from build123d import *

# Parameters (mm, degrees)
BOSS_EXTRUDE1_DEPTH                       = 3.175
CSK_FOR_0_FLAT_HEAD_MACHINE_SCREW_2_COUNT = 2
CSK_FOR_0_FLAT_HEAD_MACHINE_SCREW_2_PITCH = 47.625
LPATTERN1_COUNT                           = 4
LPATTERN1_PITCH                           = 25.4
LPATTERN2_COUNT                           = 3
LPATTERN2_PITCH                           = 50.8


with BuildPart() as part:
    # Sketch1 → Boss-Extrude1 (new body)
    with BuildSketch(Plane.XY):
        with BuildLine():
            Line((0, 0), (0, 220.98))
            Line((0, 220.98), (-6.35, 220.98))
            ThreePointArc((-6.35, 220.98), (-10.840128061, 222.839871939), (-12.7, 227.33))
            Line((-12.7, 227.33), (-12.7, 284.48))
            Line((-12.7, 284.48), (-129.54, 284.48))
            Line((-129.54, 284.48), (-129.54, 227.33))
            Line((-129.54, 227.33), (-44.45, 0))
            Line((-44.45, 0), (0, 0))
        make_face()
    extrude(amount=-BOSS_EXTRUDE1_DEPTH)

    # Sketch3 → CSK for _0 Flat Head Machine Screw _100 (revolve, cut)
    with BuildSketch(Plane(origin=(-114.3, 278.13, 0), x_dir=(0, -1, 0), z_dir=(1, 0, 0))):
        Polygon((0, 0), (0, 3.175), (2.7559, 3.175), (2.7559, 2.4384), (5.1943, 0), align=None)
    csk_for_0_flat_head_machine_screw_100 = revolve(axis=Axis((-114.3, 278.13, 6.35), (0, 0, -1)), mode=Mode.SUBTRACT)

    # CSK for _0 Flat Head Machine Screw _ 2: CSK for _0 Flat Head Machine Screw _100 ×2
    with Locations(*[(0, -i * CSK_FOR_0_FLAT_HEAD_MACHINE_SCREW_2_PITCH, 0) for i in range(1, CSK_FOR_0_FLAT_HEAD_MACHINE_SCREW_2_COUNT)]):
        add(csk_for_0_flat_head_machine_screw_100, mode=Mode.SUBTRACT)

    # LPattern1: CSK for _0 Flat Head Machine Screw _100 ×4
    with Locations(*[(i * LPATTERN1_PITCH, 0, 0) for i in range(1, LPATTERN1_COUNT)]):
        add(csk_for_0_flat_head_machine_screw_100, mode=Mode.SUBTRACT)

    # LPattern1 copy 1 sketch → LPattern1 copy 1 (revolve, cut)
    with BuildSketch(Plane(origin=(-88.9, 230.505, 0), x_dir=(0, -1, 0), z_dir=(1, 0, 0))):
        Polygon((0, 0), (0, 3.175), (2.7559, 3.175), (2.7559, 2.4384), (5.1943, 0), align=None)
    revolve(axis=Axis((-88.9, 230.505, 6.35), (0, 0, -1)), mode=Mode.SUBTRACT)

    # LPattern1 copy 2 sketch → LPattern1 copy 2 (revolve, cut)
    with BuildSketch(Plane(origin=(-63.5, 230.505, 0), x_dir=(0, -1, 0), z_dir=(1, 0, 0))):
        Polygon((0, 0), (0, 3.175), (2.7559, 3.175), (2.7559, 2.4384), (5.1943, 0), align=None)
    revolve(axis=Axis((-63.5, 230.505, 6.35), (0, 0, -1)), mode=Mode.SUBTRACT)

    # LPattern1 copy 3 sketch → LPattern1 copy 3 (revolve, cut)
    with BuildSketch(Plane(origin=(-38.1, 230.505, 0), x_dir=(0, -1, 0), z_dir=(1, 0, 0))):
        Polygon((0, 0), (0, 3.175), (2.7559, 3.175), (2.7559, 2.4384), (5.1943, 0), align=None)
    revolve(axis=Axis((-38.1, 230.505, 6.35), (0, 0, -1)), mode=Mode.SUBTRACT)

    # Sketch4 → CSK for _0 Flat Head Machine Screw _ 3 (revolve, cut)
    with BuildSketch(Plane(origin=(-15.875, 107.95, 0), x_dir=(0, -1, 0), z_dir=(1, 0, 0))):
        Polygon((0, 0), (0, 3.175), (2.7559, 3.175), (2.7559, 2.4384), (5.1943, 0), align=None)
    csk_for_0_flat_head_machine_screw_3 = revolve(axis=Axis((-15.875, 107.95, 6.35), (0, 0, -1)), mode=Mode.SUBTRACT)

    # LPattern2: CSK for _0 Flat Head Machine Screw _ 3 ×3
    with Locations(*[(0, -i * LPATTERN2_PITCH, 0) for i in range(1, LPATTERN2_COUNT)]):
        add(csk_for_0_flat_head_machine_screw_3, mode=Mode.SUBTRACT)


solid = part.part
The listing builds one solid part. Answer for the finished solid, in the listing's coordinates (mm). Round coordinates to 2 decimals unless told otherwise and drop trailing zeros. Write each loop counter-clockwise with the first axis right and the second up, starting at its lowest first coordinate (ties: lowest second). Pieces come first, ordered by that corner, then holes. Notation, with made-up numbers: (32, -22) - (67, -22) arc R35 cw to (67, 14) - close; hole circle Ø10 at (-16.5, 39). An arc over 180 degrees is marked (long way). Use a Markdown table: item, result. Add a question column.
1. The part is cut by section C-C (y = 6.35). Write down the section's boundary in (x, z) (3 decimals).
2. The part is cut by section A-A (y = 278.13). Write down the section's boundary in (x, z) (3 decimals), and give its area (3 significant figures).
3. The part is cut by section B-B (x = -38.1). Write down the section's boundary in (y, z) (3 decimals), and give its area (3 significant figures).
4. Flat-ended cylindrical pins translate along their axes: P1, Ø6.5, axis at x = -63.5, y = 230.505, coming from the -Z side (3 decimals); P2, Ø4.5, axis at x = -114.3, y = 230.505, coming from the -Z side; P3, Ø9, axis at x = -114.3, y = 278.13, coming from the +Z side; P4, Ø1, axis at x = -4, z = -1.5, coming from the +Y side. Find the tip coordinate at first contact, or state that the pin passes through.
5. Consider line 1 (X direction, y = 278.13, z = -2.65); line 2 (X direction, y = 228, z = -0.5); line 3 (X direction, y = 234.5, z = -2). Determine where each line is inside the solid, lowest interval first.
6. The part is cut by section D-D (z = -1.55). Give the number of separate pieces and of enclosed holes in the cut face, and give its area (3 significant figures).
7. For a pull along Y with two mould halves and no side action, classify faces 1 (the face through (-38.221, 280.883, -2.802)), 2 (the face through (-10.8, 222.8, -1.6)), 3 (the face through (-87.59, 115.26, -1.57)) as +Y half, -Y half, draft (parallel to the pull), parting line (faces both ways), or undercut.
Reported:
| question | item | result |
|---|---|---|
| 1 | outline | (-46.827, -3.175) - (-18.631, -3.175) - (-18.631, -2.438) - (-21.069, 0) - (-46.827, 0) - close; (-13.119, -3.175) - (0, -3.175) - (0, 0) - (-10.681, 0) - (-13.119, -2.438) - close |
| 2 | outline | (-129.54, -3.175) - (-117.056, -3.175) - (-117.056, -2.438) - (-119.494, 0) - (-129.54, 0) - close; (-111.544, -3.175) - (-91.656, -3.175) - (-91.656, -2.438) - (-94.094, 0) - (-109.106, 0) - (-111.544, -2.438) - close; (-86.144, -3.175) - (-66.256, -3.175) - (-66.256, -2.438) - (-68.694, 0) - (-83.706, 0) - (-86.144, -2.438) - close; (-60.744, -3.175) - (-40.856, -3.175) - (-40.856, -2.438) - (-43.294, 0) - (-58.306, 0) - (-60.744, -2.438) - close; (-35.344, -3.175) - (-12.7, -3.175) - (-12.7, 0) - (-32.906, 0) - (-35.344, -2.438) - close |
| 2 | area | 277 mm^2 |
| 3 | outline | (0, -3.175) - (227.749, -3.175) - (227.749, -2.438) - (225.311, 0) - (0, 0) - close; (233.261, -3.175) - (275.374, -3.175) - (275.374, -2.438) - (272.936, 0) - (235.699, 0) - (233.261, -2.438) - close; (280.886, -3.175) - (284.48, -3.175) - (284.48, 0) - (283.324, 0) - (280.886, -2.438) - close |
| 3 | area | 856 mm^2 |
| 4 | P1 | z = -3.175 |
| 4 | P2 | through |
| 4 | P3 | z = -0.69 |
| 4 | P4 | y = 220.98 |
| 5 | line 1 | -129.54 to -117.06, -111.54 to -91.66, -86.14 to -66.26, -60.74 to -40.86, -35.34 to -12.7 |
| 5 | line 2 | -129.54 to -118.27, -110.33 to -92.87, -84.93 to -67.47, -59.53 to -42.07, -34.13 to -12.7 |
| 5 | line 3 | -129.54 to -12.7 |
| 6 | separate pieces | 1 |
| 6 | enclosed holes | 11 |
| 6 | area | 25,900 mm^2 |
| 7 | face 1 | undercut |
| 7 | face 2 | +Y half |
| 7 | face 3 | -Y half |
